```python
from build123d import *

# Parameters (mm, degrees)
ESQUISSE1_W           = 150
ESQUISSE1_H           = 200
EXTRUSION1_DEPTH      = 22
ESQUISSE2_R           = 4.5
EXTRUSION2_DEPTH      = 30
EXTRUSION2_DEPTH_BACK = 160


with BuildPart() as part:
    # Esquisse1 → Extrusion1 (new body)
    with BuildSketch(Plane.XY):
        with Locations((75, 100)):
            Rectangle(ESQUISSE1_W, ESQUISSE1_H)
    extrude(amount=EXTRUSION1_DEPTH)

    # Esquisse2 → Extrusion2 (add, two sides)
    with BuildSketch(Plane.ZY) as extrusion2_sk:
        with Locations((11, 15)):
            Circle(ESQUISSE2_R)
    extrude(amount=EXTRUSION2_DEPTH)
    extrude(extrusion2_sk.sketch, amount=-EXTRUSION2_DEPTH_BACK)


solid = part.part
```
Build history of the part. All positions in model axes, mm. A direction names the side the tool comes from. Round coordinates to 2 decimals unless told otherwise and drop trailing zeros. Write each loop counter-clockwise with the first axis right and the second up, starting at its lowest first coordinate (ties: lowest second). Pieces come first, ordered by that corner, then holes. Notation, with made-up numbers: (36, -17.5) - (95, -17.5) arc R11 ccw to (95, -11.5) - close; hole circle Ø8 at (40, 28). An arc over 180 degrees is marked (long way). Write each question's results on one line, items separated by ' | '. Start each with the question number.
Item 1: Which spindle directions (+Z, -Z, +X, -X, +Y, -Y) get a long thin tool onto all of the face, cutting with end or side? Do faces 1 (the face through (-30, 15, 11)), 2 (the face through (154.93, 18.794, 13.419)), 3 (the face through (-14.79, 18.794, 13.419)). Say none if no direction does.
Item 2: Drop flat-ended pins along their axis: P1, Ø3, axis at y = 54.5, z = 9, coming from the +X side; P2, Ø12, axis at x = 127.5, y = 140.5, coming from the -Z side; P3, Ø8, axis at y = 152, z = 3.5, coming from the -X side. Give the stop position or say it passes through.
Item 3: Saw through at D-D (y = 75.5). Write the cut outline in (x, z), and give its area (3 significant figures).
Item 4: Saw through at B-B (z = 11). Write the cut outline in (x, y), and give its area (3 significant figures).
Item 5: Wall check: L1, parallel to X at y = 63, z = 9.75. Give the ranges that are in metal, low to high. Write a range as [from, to].
Item 6: Saw through at A-A (y = 15). Write the cut outline in (x, z), and give its area (3 significant figures).
Item 7: Saw through at C-C (x = -5). Write the cut outline in (y, z), and give its area (3 significant figures).
Results are:
1) face 1: +Z, -Z, -X, +Y, -Y | face 2: +X | face 3: -X
2) P1: stops at x = 150 | P2: stops at z = 0 | P3: stops at x = 0
3) outline: (0, 0) - (150, 0) - (150, 22) - (0, 22) - close | area: 3,300 mm²
4) outline: (-30, 10.5) - (0, 10.5) - (0, 0) - (150, 0) - (150, 10.5) - (160, 10.5) - (160, 19.5) - (150, 19.5) - (150, 200) - (0, 200) - (0, 19.5) - (-30, 19.5) - close | area: 30,400 mm²
5) L1: x = [0, 150]
6) outline: (-30, 6.5) - (0, 6.5) - (0, 0) - (150, 0) - (150, 6.5) - (160, 6.5) - (160, 15.5) - (150, 15.5) - (150, 22) - (0, 22) - (0, 15.5) - (-30, 15.5) - close | area: 3,660 mm²
7) outline: circle Ø9 at (15, 11) | area: 63.6 mm²
